```python
from build123d import *
from build123d.topology import SkipClean

# Parameters (mm, degrees)
SKETCH_1_R      = 5.02
SKETCH_1_R_2    = 0.95
EXTRUDE_1_DEPTH = 4.4
EXTRUDE_START   = 0.4
SKETCH_3_R      = 5.62
SKETCH_3_R_2    = 0.95
EXTRUDE_2_DEPTH = 0.4
CHAMFER_1_SIZE  = 0.5


with BuildPart() as part:
    # 草图1 → 凸台-拉伸1 (new body)
    with BuildSketch(Plane(origin=(0, 0, 0), x_dir=(1, 0, 0), z_dir=(0, 1, 0))):
        with Locations(Location((0, 0, 0), (0, 0, 270))):
            Circle(SKETCH_1_R)
        with Locations(Location((3.2, 0, 0), (0, 0, 270))):
            Circle(SKETCH_1_R_2, mode=Mode.SUBTRACT)
        with Locations(Location((-0.8, 0, 0), (0, 0, 90))):
            Circle(SKETCH_1_R_2, mode=Mode.SUBTRACT)
    extrude(amount=EXTRUDE_1_DEPTH)

    # 草图3 → 凸台-拉伸2 (add)
    with SkipClean():  # the faces are left unmerged after this step: merging them gives an invalid solid
        with BuildSketch(Plane.XZ.offset(EXTRUDE_START)):
            with Locations(Location((0, 0, 0), (0, 0, 270))):
                Circle(SKETCH_3_R)
            with Locations(Location((3.2, 0, 0), (0, 0, 270))):
                Circle(SKETCH_3_R_2, mode=Mode.SUBTRACT)
            with Locations(Location((-0.8, 0, 0), (0, 0, 270))):
                Circle(SKETCH_3_R_2, mode=Mode.SUBTRACT)
        extrude(amount=-EXTRUDE_2_DEPTH)

    # 倒角1
    # the kernel refuses this chamfer: 0.5 mm, written as the material it takes off along each edge
    with BuildSketch(Plane(origin=(3.2, -0.4, 0), x_dir=(0, 0, -1), z_dir=(-1, 0, 0))) as chamfer_1_piece_1:
        Polygon((0.95 + CHAMFER_1_SIZE, 0), (0.95, -CHAMFER_1_SIZE), (0.95, 0), align=None)
    revolve(axis=Axis((3.2, -0.4, 0), (0, -1, 0)), mode=Mode.SUBTRACT)
    with BuildSketch(Plane(origin=(-0.8, -0.4, 0), x_dir=(0, 0, -1), z_dir=(-1, 0, 0))) as chamfer_1_piece_2:
        Polygon((0.95 + CHAMFER_1_SIZE, 0), (0.95, -CHAMFER_1_SIZE), (0.95, 0), align=None)
    revolve(axis=Axis((-0.8, -0.4, 0), (0, -1, 0)), mode=Mode.SUBTRACT)
    with BuildSketch(Plane(origin=(0, 4.4, 0), x_dir=(0, 0, 1), z_dir=(-1, 0, 0))) as chamfer_1_piece_3:
        Polygon((5.02, -CHAMFER_1_SIZE), (5.02 - CHAMFER_1_SIZE, 0), (5.02, 0), align=None)
    revolve(axis=Axis((0, 4.4, 0), (0, 1, 0)), mode=Mode.SUBTRACT)
    with BuildSketch(Plane(origin=(3.2, 4.4, 0), x_dir=(0, 0, 1), z_dir=(-1, 0, 0))) as chamfer_1_piece_4:
        Polygon((0.95 + CHAMFER_1_SIZE, 0), (0.95, -CHAMFER_1_SIZE), (0.95, 0), align=None)
    revolve(axis=Axis((3.2, 4.4, 0), (0, 1, 0)), mode=Mode.SUBTRACT)
    with BuildSketch(Plane(origin=(-0.8, 4.4, 0), x_dir=(0, 0, -1), z_dir=(1, 0, 0))) as chamfer_1_piece_5:
        Polygon((0.95 + CHAMFER_1_SIZE, 0), (0.95, -CHAMFER_1_SIZE), (0.95, 0), align=None)
    revolve(axis=Axis((-0.8, 4.4, 0), (0, 1, 0)), mode=Mode.SUBTRACT)


solid = part.part
```
The listing builds one solid part. Answer for the finished solid, in the listing's coordinates (mm). A direction names the side the tool comes from. Give positions to 0.01 mm unless a question says otherwise; leave off trailing zeros. Loops run counter-clockwise (first coordinate to the right, second up) from the corner with the lowest first, then second, coordinate; pieces in that order, holes last. Notation, with made-up numbers: (14, 16) - (19, 16) arc R33 ccw to (19, 53) - close; hole circle Ø9 at (3, 45.25). An arc over 180 degrees is marked (long way). Answer as CSV lines item,"result". Start each with the question number.
Item 1: A cutting plane is placed at C-C on z = 5.25. Determine the outline of the cut face in (x, y), then the cut area to 3 significant figures.
Item 2: Each of these flat-tipped pins is pushed along its axis until it touches: pin 1 (1.5 mm diameter, centred on x = 3.2, z = 0, fed in from +Y); pin 2 (1 mm diameter, centred on x = -4, y = 1, fed in from -Z); pin 3 (1.5 mm diameter, centred on x = -4.5, y = 3, fed in from -Z). Where does it stop, or does it pass through?
Item 3: A cutting plane is placed at A-A on z = 0. Determine the outline of the cut face in (x, y) (3 decimals), then the cut area to 3 significant figures.
Item 4: For faces 1 (the face through (2.273, 1.973, -0.206)), 2 (the face through (5, 0, 2)), determine the directions among +Z, -Z, +X, -X, +Y, -Y from which every point of the face is accessible in a straight line to the end or side of a thin tool.
Item 5: A cutting plane is placed at B-B on y = 1.55. Determine the outline of the cut face in (x, z).
Item 6: The mould has two halves that part along Z. Classify faces 3 (the face through (0.127, 1.973, 0.206)), 4 (the face through (1.508, 1.923, 4.788)), 5 (the face through (1, -0.4, 0)): +Z half, -Z half, draft (parallel to the pull), parting line (faces both ways), or undercut.
Item 7: Find the intervals of material crossed by line 1 (X direction, y = 2.6, z = 0); line 2 (X direction, y = 3, z = 0.5); line 3 (Z direction, x = 2.5, y = 2.05), in increasing order. Write a range as from..to.
Found:
1,outline,"(-2.01, -0.4) - (2.01, -0.4) - (2.01, 0) - (-2.01, 0) - close"
1,area,"1.60 mm^2"
2,pin 1,"passes through"
2,pin 2,"stops at z = -3.6"
2,pin 3,"stops at z = -3.34"
3,outline,"(-5.62, -0.4) - (-2.25, -0.4) - (-1.75, 0.1) - (-1.75, 3.9) - (-2.25, 4.4) - (-4.52, 4.4) - (-5.02, 3.9) - (-5.02, 0) - (-5.62, 0) - close; (0.15, 0.1) - (0.65, -0.4) - (1.75, -0.4) - (2.25, 0.1) - (2.25, 3.9) - (1.75, 4.4) - (0.65, 4.4) - (0.15, 3.9) - close; (4.15, 0.1) - (4.65, -0.4) - (5.62, -0.4) - (5.62, 0) - (5.02, 0) - (5.02, 3.9) - (4.585, 4.335) - (4.15, 3.9) - close"
3,area,"29.2 mm^2"
4,face 1,"+Y, -Y"
4,face 2,"+Y"
5,outline,"circle Ø10.04 at (0, 0); hole circle Ø1.9 at (-0.8, 0); hole circle Ø1.9 at (3.2, 0)"
6,face 3,"undercut"
6,face 4,"parting line"
6,face 5,"draft"
7,line 1,"x = -5.02..-1.75, 0.15..2.25, 4.15..5.02"
7,line 2,"x = -5..-1.61, 0.01..2.39, 4.01..5"
7,line 3,"z = -4.35..-0.64, 0.64..4.35"
